Read the model definition and answer for the solid it produces. Units are mm, in the model's axes. Give positions to 0.01 mm unless a question says otherwise; leave off trailing zeros. Loops run counter-clockwise (first coordinate to the right, second up) from the corner with the lowest first, then second, coordinate; pieces in that order, holes last.
(1) Each of these flat-tipped pins is pushed along its axis until it touches: P1, Ø1.5, axis at x = 2.5, z = -13, coming from the -Y side; P2, Ø6, axis at x = -6.5, y = 34.5, coming from the +Z side; P3, Ø2, axis at x = 4, z = 5, coming from the -Y side; P4, Ø2, axis at x = -7.5, y = 26.5, coming from the +Z side. Where does it stop, or does it pass through?
(2) Determine the mould class of faces 1 (the face through (0.161, 48.595, -13.67)), 2 (the face through (-11.5, 30, -10)), 3 (the face through (0.253, 29.58, 11.497)) for opening direction Z: pulls with the +Z half, pulls with the -Z half, needs draft (parallel to the pull), parting line crosses it, or undercut.
(3) Find section A-A, the plane y = 9.5. Write down the section's boundary in (x, z).
(4) Find section C-C, the plane z = -17. Write down the section's boundary in (x, y), then the cut area to 3 significant figures.
(5) Find section D-D, the plane y = 42. Write down the section's boundary in (x, z), then the cut area to 3 significant figures.
(6) Straight lines are drawn through the part: probe 1 along Y at (x, z) = (-9, -16); probe 2 along Y at (x, z) = (-6.5, -14); probe 3 along Z at (x, y) = (-1.5, 15.5). For each, find the intervals that lie inside material, in ascending order.
(7) Find section B-B, the plane x = 4. Write down the section's boundary in (y, z), then the cut area to 3 significant figures.
```python
from build123d import *

# Parameters (mm, degrees)
SKETCH1_R           = 7.5
BOSS_EXTRUDE1_DEPTH = 60
SKETCH2_R           = 4
CUT_EXTRUDE1_DEPTH  = 50


with BuildPart() as part:
    # Sketch1 → Boss-Extrude1 (new body)
    with BuildSketch(Plane(origin=(0, 0, 0), x_dir=(1, 0, 0), z_dir=(0, 1, 0))):
        with BuildLine():
            Line((-11.5, 0), (-11.5, 20.793359223))
            Line((-11.5, 20.793359223), (11.5, 20.793359223))
            Line((11.5, 20.793359223), (11.5, 0))
            ThreePointArc((11.5, 0), (0, -11.5), (-11.5, 0))
        make_face()
        with Locations(Location((0, 0, 0), (0, 0, 270))):
            Circle(SKETCH1_R, mode=Mode.SUBTRACT)
    extrude(amount=BOSS_EXTRUDE1_DEPTH)

    # Sketch2 → Cut-Extrude1 (cut)
    with BuildSketch(Plane(origin=(11.5, 0, 0), x_dir=(0, 0, -1), z_dir=(1, 0, 0))):
        with Locations((14.537325079, 52.5)):
            Circle(SKETCH2_R)
        with Locations((14.537325079, 7.5)):
            Circle(SKETCH2_R)
    extrude(amount=-CUT_EXTRUDE1_DEPTH, mode=Mode.SUBTRACT)


solid = part.part
```
Entries:
1. P1: stops at y = 0
1. P2: stops at z = 10.95
1. P3: passes through
1. P4: stops at z = 9.49
2. face 1: undercut
2. face 2: needs draft
2. face 3: pulls with the +Z half
3. outline: (-11.5, -20.79) - (11.5, -20.79) - (11.5, -18) - (-11.5, -18) - close; (-11.5, -11.07) - (11.5, -11.07) - (11.5, 0) arc R11.5 ccw to (-11.5, 0) - close; hole circle Ø15 at (0, 0)
4. outline: (-11.5, 0) - (11.5, 0) - (11.5, 4.35) - (-11.5, 4.35) - close; (-11.5, 10.65) - (11.5, 10.65) - (11.5, 49.35) - (-11.5, 49.35) - close; (-11.5, 55.65) - (11.5, 55.65) - (11.5, 60) - (-11.5, 60) - close
4. area: 1,090 mm2
5. outline: (-11.5, -20.79) - (11.5, -20.79) - (11.5, 0) arc R11.5 ccw to (-11.5, 0) - close; hole circle Ø15 at (0, 0)
5. area: 509 mm2
6. probe 1: y = 0 to 3.78, 11.22 to 48.78, 56.22 to 60
6. probe 2: y = 0 to 3.54, 11.46 to 48.54, 56.46 to 60
6. probe 3: z = -20.79 to -7.35, 7.35 to 11.4
7. outline: (0, -20.79) - (60, -20.79) - (60, -6.34) - (0, -6.34) - close; (0, 6.34) - (60, 6.34) - (60, 10.78) - (0, 10.78) - close; hole circle Ø8 at (7.5, -14.54); hole circle Ø8 at (52.5, -14.54)
7. area: 1,030 mm2
